from build123d import *

# Parameters (mm, degrees)
SKETCH2_W            = 300
SKETCH2_H            = 180
BOSS_EXTRUDE1_DEPTH  = 50
CUT_EXTRUDE1_DEPTH   = 15
BOSS_EXTRUDE4_DEPTH  = 50
SKETCH10_W           = 105
SKETCH10_H           = 180
BOSS_EXTRUDE7_DEPTH  = 50
CUT_EXTRUDE3_DEPTH   = 105
CUT_EXTRUDE4_DEPTH   = 15
SKETCH14_W           = 70
SKETCH14_H           = 65
SKETCH14_W_2         = 95
BOSS_EXTRUDE8_DEPTH  = 35
CUT_EXTRUDE5_DEPTH   = 195
SHELL1_T             = -10
SKETCH16_W           = 21
SKETCH16_H           = 46
CUT_EXTRUDE7_DEPTH   = 10
SKETCH17_R           = 17.5
CUT_EXTRUDE15_DEPTH  = 10
CUT_EXTRUDE16_DEPTH  = 10
SKETCH22_W           = 40.092518347
SKETCH22_H           = 11.168807906
CUT_EXTRUDE17_DEPTH  = 33
SKETCH23_W           = 21
SKETCH23_H           = 10
BOSS_EXTRUDE9_DEPTH  = 3
SKETCH24_W           = 21
SKETCH24_H           = 3
BOSS_EXTRUDE10_DEPTH = 5
CUT_EXTRUDE18_DEPTH  = 10
SKETCH27_W           = 26
SKETCH27_H           = 30
CUT_EXTRUDE19_DEPTH  = 10


with BuildPart() as part:
    # Sketch2 → Boss-Extrude1 (new body)
    with BuildSketch(Plane(origin=(0, 0, 0), x_dir=(1, 0, 0), z_dir=(0, 1, 0))):
        with Locations((150, 90)):
            Rectangle(SKETCH2_W, SKETCH2_H)
    extrude(amount=BOSS_EXTRUDE1_DEPTH)

    # Sketch3 → Cut-Extrude1 (cut)
    with BuildSketch(Plane(origin=(0, 50, 0), x_dir=(1, 0, 0), z_dir=(0, 1, 0))):
        with BuildLine():
            Line((90, 12), (90, 73))
            ThreePointArc((90, 73), (90.585786438, 74.414213562), (92, 75))
            Line((92, 75), (183, 75))
            ThreePointArc((183, 75), (184.414213562, 74.414213562), (185, 73))
            Line((185, 73), (185, 12))
            ThreePointArc((185, 12), (184.414213562, 10.585786438), (183, 10))
            Line((183, 10), (92, 10))
            ThreePointArc((92, 10), (90.585786438, 10.585786438), (90, 12))
        make_face()
        with BuildLine():
            Line((12, 10), (78, 10))
            ThreePointArc((78, 10), (79.414213562, 10.585786438), (80, 12))
            Line((80, 12), (80, 73))
            ThreePointArc((80, 73), (79.414213562, 74.414213562), (78, 75))
            Line((78, 75), (12, 75))
            ThreePointArc((12, 75), (10.585786438, 74.414213562), (10, 73))
            Line((10, 73), (10, 12))
            ThreePointArc((10, 12), (10.585786438, 10.585786438), (12, 10))
        make_face()
    extrude(amount=-CUT_EXTRUDE1_DEPTH, mode=Mode.SUBTRACT)

    # Sketch6 → Boss-Extrude4 (add)
    with BuildSketch(Plane(origin=(0, 50, 0), x_dir=(1, 0, 0), z_dir=(0, 1, 0))):
        Polygon((0, 180), (185, 180), (195, 180), (195, 95), (185, 95), (0, 95), align=None)
        with BuildLine():
            Line((185, 168), (185, 107))
            ThreePointArc((185, 107), (184.414213562, 105.585786438), (183, 105))
            Line((183, 105), (92, 105))
            ThreePointArc((92, 105), (90.585786438, 105.585786438), (90, 107))
            Line((90, 107), (90, 168))
            ThreePointArc((90, 168), (90.585786438, 169.414213562), (92, 170))
            Line((92, 170), (183, 170))
            ThreePointArc((183, 170), (184.414213562, 169.414213562), (185, 168))
        make_face(mode=Mode.SUBTRACT)
        with BuildLine():
            Line((80, 107), (80, 168))
            ThreePointArc((80, 168), (79.414213562, 169.414213562), (78, 170))
            Line((78, 170), (12, 170))
            ThreePointArc((12, 170), (10.585786438, 169.414213562), (10, 168))
            Line((10, 168), (10, 107))
            ThreePointArc((10, 107), (10.585786438, 105.585786438), (12, 105))
            Line((12, 105), (78, 105))
            ThreePointArc((78, 105), (79.414213562, 105.585786438), (80, 107))
        make_face(mode=Mode.SUBTRACT)
    extrude(amount=BOSS_EXTRUDE4_DEPTH)

    # Sketch10 → Boss-Extrude7 (add)
    with BuildSketch(Plane(origin=(0, 50, 0), x_dir=(1, 0, 0), z_dir=(0, 1, 0))):
        with Locations((247.5, 90)):
            Rectangle(SKETCH10_W, SKETCH10_H)
    extrude(amount=BOSS_EXTRUDE7_DEPTH)

    # Sketch11 → Cut-Extrude3 (cut)
    with BuildSketch(Plane(origin=(300, 0, 0), x_dir=(0, 0, -1), z_dir=(1, 0, 0))):
        Polygon((0, 100), (180, 100), (0, 50), align=None)
    extrude(amount=-CUT_EXTRUDE3_DEPTH, mode=Mode.SUBTRACT)

    # Sketch13 → Cut-Extrude4 (cut)
    with BuildSketch(Plane(origin=(0, 46.418338109, 12.893982808), x_dir=(1, 0, 0), z_dir=(0, 0.9635179096299407, 0.2676438637860946))):
        with BuildLine():
            Line((288, 190.197610112), (207, 190.197610112))
            ThreePointArc((207, 190.197610112), (205.585786438, 189.611823674), (205, 188.197610112))
            Line((205, 188.197610112), (205, 25.382193189))
            ThreePointArc((205, 25.382193189), (205.585786438, 23.967979627), (207, 23.382193189))
            Line((207, 23.382193189), (288, 23.382193189))
            ThreePointArc((288, 23.382193189), (289.414213562, 23.967979627), (290, 25.382193189))
            Line((290, 25.382193189), (290, 188.197610112))
            ThreePointArc((290, 188.197610112), (289.414213562, 189.611823674), (288, 190.197610112))
        make_face()
    extrude(amount=-CUT_EXTRUDE4_DEPTH, mode=Mode.SUBTRACT)

    # Sketch14 → Boss-Extrude8 (add)
    with BuildSketch(Plane(origin=(0, 50, 0), x_dir=(1, 0, 0), z_dir=(0, 1, 0))):
        with Locations((45, 137.5)):
            Rectangle(SKETCH14_W, SKETCH14_H)
        with Locations((137.5, 137.5)):
            Rectangle(SKETCH14_W_2, SKETCH14_H)
    extrude(amount=BOSS_EXTRUDE8_DEPTH)

    # Sketch15 → Cut-Extrude5 (cut)
    with BuildSketch(Plane.ZY):
        Polygon((-180, 0), (0, 0), (0, 50), (-95, 50), (-95, 100), (-180, 100), align=None)
    extrude(amount=-CUT_EXTRUDE5_DEPTH, mode=Mode.SUBTRACT)

    # Shell1
    shell1_openings = [part.faces().sort_by_distance(p)[0] for p in [
        (247.5, 0, -90),
    ]]
    offset(amount=SHELL1_T, openings=shell1_openings, kind=Kind.INTERSECTION)

    # Sketch16 → Cut-Extrude7 (cut)
    with BuildSketch(Plane(origin=(0, 31.965569464, 8.879324851), x_dir=(1, 0, 0), z_dir=(0, 0.9635179096299407, 0.2676438637860946))):
        with Locations((247.5, 106.782193189)):
            Rectangle(SKETCH16_W, SKETCH16_H)
    extrude(amount=-CUT_EXTRUDE7_DEPTH, mode=Mode.SUBTRACT)

    # Sketch17 → Cut-Extrude15 (cut)
    with BuildSketch(Plane.ZY.offset(-195)):
        with Locations((-132.5, 25.5)):
            Circle(SKETCH17_R)
        with Locations((-47.5, 25.5)):
            Circle(SKETCH17_R)
    extrude(amount=-CUT_EXTRUDE15_DEPTH, mode=Mode.SUBTRACT)

    # Sketch20 → Cut-Extrude16 (cut)
    with BuildSketch(Plane.XY):
        Polygon((264, 38), (245, 38), (237, 38), (231, 38), (231, 34), (231, 25), (231, 5), (264, 5), align=None)
    extrude(amount=-CUT_EXTRUDE16_DEPTH, mode=Mode.SUBTRACT)

    # Sketch22 → Cut-Extrude17 (cut)
    with BuildSketch(Plane.ZY.offset(-264)):
        with Locations((-30.046259174, 32.415596047)):
            Rectangle(SKETCH22_W, SKETCH22_H)
    extrude(amount=CUT_EXTRUDE17_DEPTH, mode=Mode.SUBTRACT)

    # Sketch23 → Boss-Extrude9 (add)
    with BuildSketch(Plane(origin=(0, 34.735407636, -125.047467489), x_dir=(1, 0, 0), z_dir=(0, -0.2676438637860946, 0.9635179096299407))):
        with Locations((247.5, 18.175895481)):
            Rectangle(SKETCH23_W, SKETCH23_H)
    boss_extrude9 = extrude(amount=-BOSS_EXTRUDE9_DEPTH)

    # Sketch24 → Boss-Extrude10 (add)
    with BuildSketch(Plane(origin=(0, 34.735407636, -125.047467489), x_dir=(1, 0, 0), z_dir=(0, -0.2676438637860946, 0.9635179096299407))):
        with Locations((247.5, 14.675895481)):
            Rectangle(SKETCH24_W, SKETCH24_H)
    boss_extrude10 = extrude(amount=BOSS_EXTRUDE10_DEPTH)

    # Mirror1: Boss-Extrude9, Boss-Extrude10 across plane
    add(boss_extrude9.mirror(Plane(origin=(0, 28.579598769, -102.886555567), x_dir=(1, 0, 0), z_dir=(0, -0.2676438637860946, 0.9635179096299407))))
    add(boss_extrude10.mirror(Plane(origin=(0, 28.579598769, -102.886555567), x_dir=(1, 0, 0), z_dir=(0, -0.2676438637860946, 0.9635179096299407))))

    # Sketch26 → Cut-Extrude18 (cut)
    with BuildSketch(Plane.ZY.offset(-195)):
        with BuildLine():
            Line((-132.5, 43), (-47.5, 43))
            ThreePointArc((-47.5, 43), (-65, 25.5), (-47.5, 8))
            Line((-47.5, 8), (-132.5, 8))
            ThreePointArc((-132.5, 8), (-115, 25.5), (-132.5, 43))
        make_face()
    extrude(amount=-CUT_EXTRUDE18_DEPTH, mode=Mode.SUBTRACT)

    # Sketch27 → Cut-Extrude19 (cut)
    with BuildSketch(Plane(origin=(0, 0, -180), x_dir=(-1, 0, 0), z_dir=(0, 0, -1))):
        with Locations((-247.5, 45)):
            Rectangle(SKETCH27_W, SKETCH27_H)
    extrude(amount=-CUT_EXTRUDE19_DEPTH, mode=Mode.SUBTRACT)


solid = part.part
Input: part model. Units: mm. Frame: model coordinates. A direction names the side the tool comes from. Give positions to 0.01 mm unless a question says otherwise; leave off trailing zeros. Loops run counter-clockwise (first coordinate to the right, second up) from the corner with the lowest first, then second, coordinate; pieces in that order, holes last. Notation, with made-up numbers: (67.25, 24.5) - (118.25, 24.5) arc R21 ccw to (118.25, 50.5) - close; hole circle Ø8 at (-4.75, 63.5). An arc over 180 degrees is marked (long way). Use CSV: the item, a comma, the result in double quotes. Start each with the question number.
Item 1: Section C-C on z = -90.5. Return loops of the section in (x, y).
Item 2: Line query: line 1 (X direction, y = 72, z = -104); line 2 (Z direction, x = 230.5, y = 8.5); line 3 (Z direction, x = 248, y = 8). Output: solid intervals per line, ascending.
Item 3: Section D-D on x = 270. Return loops of the section in (y, z), then the cut area to 3 significant figures.
Item 4: Section B-B on z = -147.5. Return loops of the section in (x, y), then the cut area to 3 significant figures.
Item 5: Mould query, pull axis Y, two halves, no side actions, for faces 4 (the flat face through (300, 38, -89)), 5 (the flat face through (260.5, 45, -175)), 6 (the flat face through (247.353, 47.178, -120.611)). Classes: pulls with the +Y half, pulls with the -Y half, needs draft (parallel to the pull), parting line crosses it, or undercut.
Item 6: Reachability of faces 1 (the cylindrical face through (199.93, 25.885, -149.996)), 2 (the flat face through (234.5, 45, -175)), 3 (the flat face through (247.35, 46.31, -74.09)) from +Z, -Z, +X, -X, +Y, -Y: full face, straight path, thin tool, end or side. Return the list, or none.
Item 7: Section A-A on x = 249. State how many separate pieces and enclosed holes the cut face has, then the cut area to 3 significant figures.
Item 8: Contact query for flat-ended pins moving along their axis: P1, Ø5, axis at x = 241.5, z = -176.5, coming from the +Y side; P2, Ø1.5, axis at x = 262, z = -127.5, coming from the -Y side; P3, Ø16.5, axis at x = 241, z = -32.5, coming from the -Y side; P4, Ø11, axis at y = 39, z = -41, coming from the -X side. Output: stop coordinate, or through.
Ans:
1,outline,"(195, 0) - (205, 0) - (205, 8) - (195, 8) - close; (195, 43) - (205, 43) - (205, 49.19) - (237, 49.19) - (237, 59.57) - (205, 59.57) - (205, 75.14) - (195, 75.14) - close; (258, 49.19) - (290, 49.19) - (290, 0) - (300, 0) - (300, 75.14) - (290, 75.14) - (290, 59.57) - (258, 59.57) - close"
2,line 1,"x = 195 to 205, 290 to 300"
2,line 2,"z = -180 to -170, -10 to 0"
2,line 3,"z = -180 to -170"
3,outline,"(0, -180) - (100, -180) - (97.32, -170.36) - (82.87, -174.38) - (38.22, -13.65) - (52.68, -9.64) - (50, 0) - (0, 0) - (0, -10) - (26.83, -10) - (71.28, -170) - (0, -170) - close"
3,area,"3,150 mm2"
4,outline,"(195, 0) - (205, 0) - (205, 16.49) - (195, 16.49) - close; (195, 34.51) - (205, 34.51) - (205, 65.03) - (290, 65.03) - (290, 0) - (300, 0) - (300, 90.97) - (290, 90.97) - (290, 75.4) - (205, 75.4) - (205, 90.97) - (195, 90.97) - close"
4,area,"2,520 mm2"
5,face 4,"needs draft"
5,face 5,"undercut"
5,face 6,"pulls with the -Y half"
6,face 1,"-X"
6,face 2,"-Z"
6,face 3,"+Y"
7,separate pieces,"4"
7,enclosed holes,"0"
7,area,"1,920 mm2"
8,P1,"stops at y = 99.72"
8,P2,"stops at y = 59.26"
8,P3,"stops at y = 38"
8,P4,"stops at x = 195"
